Can you work these out from the model? Positions are in its coordinate system, mm. A direction names the side the tool comes from. Coordinates: 2 decimals unless noted, no trailing zeros. Loops run counter-clockwise (first coordinate to the right, second up) from the corner with the lowest first, then second, coordinate; pieces in that order, holes last.
```python
from build123d import *

# Parameters (mm, degrees)
SKETCH1_R               = 15.875
EXTRUDE1_DEPTH          = 50
SKETCH2_R               = 50
EXTRUDE2_DEPTH          = 10
SKETCH2_3_R             = 7.5
EXTRUDE3_DEPTH          = 50.001
EXTRUDE4_DEPTH          = 3
EXTRUDE4_DEPTH_BACK     = 43
SKETCH6_4_R             = 4
CUT_EXTRUDE1_DEPTH      = 31
CUT_EXTRUDE1_DEPTH_BACK = 71
CUT_EXTRUDE2_DEPTH      = 51.0010001
SKETCH1_3_R             = 15.875
CUT_EXTRUDE3_DEPTH      = 51.0000001
CUT_EXTRUDE3_DEPTH_BACK = 51.0000001


with BuildPart() as part:
    # Sketch1 → Extrude1 (new body, symmetric)
    with BuildSketch(Plane.XY):
        with BuildLine():
            Line((20, 0), (20, 30))
            ThreePointArc((20, 30), (0, 50), (-20, 30))
            Line((-20, 30), (-20, 0))
            Line((-20, 0), (20, 0))
        make_face()
        with Locations((0, 30)):
            Circle(SKETCH1_R, mode=Mode.SUBTRACT)
        with Locations((0, 30)):
            Circle(SKETCH1_R)
    extrude(amount=EXTRUDE1_DEPTH, both=True)

    # Sketch2 → Extrude2 (add)
    with BuildSketch(Plane.XZ):
        Circle(SKETCH2_R)
    extrude(amount=-EXTRUDE2_DEPTH)

    # Sketch2_3 → Extrude3 (add)
    with BuildSketch(Plane.XZ):
        with Locations(Location((-20, 0, 0), (0, 0, 270))):  # turned: the seam where the file's is
            Circle(SKETCH2_3_R)
        with Locations(Location((20, 0, 0), (0, 0, 270))):  # turned: the seam where the file's is
            Circle(SKETCH2_3_R)
    extrude(amount=-EXTRUDE3_DEPTH)

    # Sketch3 → Extrude4 (add, two sides)
    with BuildSketch(Plane(origin=(20, 0, 0), x_dir=(0, 0, -1), z_dir=(1, 0, 0))) as extrude4_sk:
        with BuildLine():
            Line((-33, 30), (-33, 10))
            Line((-33, 10), (-17, 10))
            Line((-17, 10), (-17, 30))
            ThreePointArc((-17, 30), (-25, 38), (-33, 30))
        make_face()
        with BuildLine():
            Line((17, 30), (17, 10))
            Line((17, 10), (33, 10))
            Line((33, 10), (33, 30))
            ThreePointArc((33, 30), (25, 38), (17, 30))
        make_face()
    extrude(amount=EXTRUDE4_DEPTH)
    extrude(extrude4_sk.sketch, amount=-EXTRUDE4_DEPTH_BACK)

    # Sketch6_4 → Cut-Extrude1 (cut, two sides)
    with BuildSketch(Plane(origin=(20, 0, 0), x_dir=(0, 0, -1), z_dir=(1, 0, 0))) as cut_extrude1_sk:
        with Locations(Location((-25, 30, 0), (0, 0, 90))):  # turned: the seam where the file's is
            Circle(SKETCH6_4_R)
        with Locations(Location((25, 30, 0), (0, 0, 90))):  # turned: the seam where the file's is
            Circle(SKETCH6_4_R)
    extrude(amount=CUT_EXTRUDE1_DEPTH, mode=Mode.SUBTRACT)
    extrude(cut_extrude1_sk.sketch, amount=-CUT_EXTRUDE1_DEPTH_BACK, mode=Mode.SUBTRACT)

    # Sketch2_4 → Cut-Extrude2 (cut, through all)
    with BuildSketch(Plane.XZ):
        with BuildLine():
            Line((20, -5), (20, 5))
            ThreePointArc((20, 5), (15, 0), (20, -5))
        make_face()
        with BuildLine():
            ThreePointArc((25, 0), (23.535533906, 3.535533906), (20, 5))
            Line((20, 5), (20, -5))
            ThreePointArc((20, -5), (23.535533906, -3.535533906), (25, 0))
        make_face()
        with BuildLine():
            Line((20, -5), (20, 5))
            ThreePointArc((20, 5), (15, 0), (20, -5))
        make_face()
        with BuildLine():
            ThreePointArc((25, 0), (23.535533906, 3.535533906), (20, 5))
            Line((20, 5), (20, -5))
            ThreePointArc((20, -5), (23.535533906, -3.535533906), (25, 0))
        make_face()
        with BuildLine():
            Line((-20, -5), (-20, 5))
            ThreePointArc((-20, 5), (-25, 0), (-20, -5))
        make_face()
        with BuildLine():
            ThreePointArc((-15, 0), (-16.464466094, 3.535533906), (-20, 5))
            Line((-20, 5), (-20, -5))
            ThreePointArc((-20, -5), (-16.464466094, -3.535533906), (-15, 0))
        make_face()
        with BuildLine():
            Line((-20, -5), (-20, 5))
            ThreePointArc((-20, 5), (-25, 0), (-20, -5))
        make_face()
        with BuildLine():
            ThreePointArc((-15, 0), (-16.464466094, 3.535533906), (-20, 5))
            Line((-20, 5), (-20, -5))
            ThreePointArc((-20, -5), (-16.464466094, -3.535533906), (-15, 0))
        make_face()
    extrude(amount=-CUT_EXTRUDE2_DEPTH, mode=Mode.SUBTRACT)

    # Sketch1_3 → Cut-Extrude3 (cut, two sides)
    with BuildSketch(Plane.XY) as cut_extrude3_sk:
        with Locations((0, 30)):
            Circle(SKETCH1_3_R)
    extrude(amount=CUT_EXTRUDE3_DEPTH, mode=Mode.SUBTRACT)
    extrude(cut_extrude3_sk.sketch, amount=-CUT_EXTRUDE3_DEPTH_BACK, mode=Mode.SUBTRACT)


solid = part.part
```
(1) If we mould it in two halves opening along Y, with no side actions, what happens to faces 5 (the cylindrical face through (19.235, 33.815, 26.201)), 6 (the cylindrical face through (-21, 38, 25)), 7 (the flat face through (-23, 21, 25))? For each: released by +Y, released by -Y, zero draft, split by the parting line, or undercut.
Check values:
face 5: undercut
face 6: released by +Y
face 7: zero draft
(2) I want a section at C-C on z = -36.5. Write out the boundary of the cut face in (x, y) (3 decimals), then the cut area to 3 significant figures.
Check values:
outline: (-34.172, 0) - (34.172, 0) - (34.172, 10) - (20, 10) - (20, 30) arc R20 ccw to (-20, 30) - (-20, 10) - (-34.172, 10) - close; hole circle Ø31.75 at (0, 30)
area: 1,320 mm2
(3) If I drill on probe 1 along X at (y, z) = (11.5, 2); probe 2 along Z at (x, y) = (-18.25, 30); probe 3 along Y at (x, z) = (0, -30) (3 decimals), over which ranges is the centre line in solid material (lowest first)?
Check values:
probe 1: x = -27.23 to -24.58, -15.42 to 15.42, 24.58 to 27.23
probe 2: z = -50 to -29, -21 to -4.68, 4.68 to 21, 29 to 50
probe 3: y = 0 to 14.125, 45.875 to 50
(4) I want a section at D-D on z = 23. Write out the boundary of the cut face in (x, y) (3 decimals), then the cut area to 3 significant figures.
Check values:
outline: (-44.396, 0) - (44.396, 0) - (44.396, 10) - (23, 10) - (23, 26.536) - (15.492, 26.536) arc R15.875 cw to (-15.492, 26.536) - (-23, 26.536) - (-23, 10) - (-44.396, 10) - close; (-23, 33.464) - (-15.492, 33.464) arc R15.875 cw to (15.492, 33.464) - (23, 33.464) - (23, 37.746) - (18.439, 37.746) arc R20 ccw to (-18.439, 37.746) - (-23, 37.746) - close
area: 1,600 mm2
(5) I'm going to push flat-ended pins straight in: pin 1 (17.5 mm diameter, centred on y = 18.5, z = -22, fed in from -X); pin 2 (3.5 mm diameter, centred on x = 22, y = 20, fed in from -Z); pin 3 (13 mm diameter, centred on y = 30, z = 25, fed in from -X). Where does each tip first touch, or does it pass through?
Check values:
pin 1: stops at x = -45.86
pin 2: stops at z = -33
pin 3: stops at x = -23
(6) Which directions (+Z, -Z, +X, -X, +Y, -Y) give clear straight access to the entire face, cutting with the end or side of a thin tool? Please do faces 1 (the flat face through (21, 20, 33)), 2 (the flat face through (-20, 19, -41)), 3 (the flat face through (-21, 20, -17)), 4 (the flat face through (-20, 19, 42)).
Check values:
face 1: +Z, +X, +Y
face 2: -Z, -X, +Y
face 3: -X, +Y
face 4: +Z, -X, +Y
(7) I want a section at A-A on x = 0. Write out the boundary of the cut face in (y, z) (3 decimals), then the cut area to 4 significant figures.
Check values:
outline: (0, -50) - (14.125, -50) - (14.125, 50) - (0, 50) - close; (45.875, -50) - (50, -50) - (50, 50) - (45.875, 50) - close
area: 1,825 mm2
(8) I want a section at B-B on y = 6. Write out the boundary of the cut face in (x, z), then the cut area to 3 significant figures.
Check values:
outline: (-20, -50) - (20, -50) - (20, -45.83) arc R50 ccw to (20, 45.83) - (20, 50) - (-20, 50) - (-20, 45.83) arc R50 ccw to (-20, -45.83) - close; hole circle Ø10 at (-20, 0); hole circle Ø10 at (20, 0)
area: 7,810 mm2
